Could you check a few things on this model? Use its own coordinates, in mm. A direction names the side the tool comes from. Round coordinates to 2 decimals unless told otherwise and drop trailing zeros. Loops run counter-clockwise (first coordinate to the right, second up) from the corner with the lowest first, then second, coordinate; pieces in that order, holes last. Notation, with made-up numbers: (22, -39) -> (39, -39) arc R13 ccw to (39, -18) -> close; hole circle Ø10 at (8, 18.5). An arc over 180 degrees is marked (long way). Put each result on its own line as item: value. Start each with the question number.
1. Which directions (+Z, -Z, +X, -X, +Y, -Y) give clear straight access to the entire face, cutting with the end or side of a thin tool? Please do faces 1 (the conical face through (-2.465, 114.221, -18.777)), 2 (the cylindrical face through (30.995, 18.783, 6.883)), 3 (the flat face through (0, 189.23, 0)).
2. I'm going to push flat-ended pins straight in: P1, Ø6, axis at y = 3, z = -4.5, coming from the +X side; P2, Ø1, axis at y = 116, z = -14.5, coming from the -X side; P3, Ø2, axis at x = -4.5, z = 21, coming from the -Y side. Where does each tip first touch, or does it pass through?
3. Imagine slicing it at A-A, the plane y = 167. Please give me the cut outline in (x, z), and give its area (3 significant figures).
4. If we mould it in two halves opening along Y, with no side actions, what happens to faces 4 (the cylindrical face through (-6.607, 23.091, 29.755)), 5 (the flat face through (0, 190.5, 0)), 6 (the flat face through (25, 38.1, 20)), 7 (the flat face through (-28.5, 39.37, 11.8))? For each: pulls with the +Y half, pulls with the -Y half, needs draft (parallel to the pull), parting line crosses it, or undercut.
5. I need wall thicknesses on line 1 (X direction, y = 26, z = 0); line 2 (Z direction, x = -12, y = 90.5). Which ranges of each line are inside material? Lowest first, please. Write a range as [from, to].
```python
from build123d import *

# Parameters (mm, degrees)
SKETCH1_R           = 31.75
BOSS_EXTRUDE1_DEPTH = 38.1
SKETCH2_R           = 33.734375
BOSS_EXTRUDE2_DEPTH = 152.4
BOSS_EXTRUDE2_TAPER = 11
FILLET1_R           = 2.794
SKETCH4_R           = 6.35
REVOLVE1_ANGLE      = 180
SKETCH5_R           = 31.75
BOSS_EXTRUDE3_DEPTH = 6.35


# Read off the part's stored shape, not the designer's step: Shell3
with BuildPart() as part:
    # Sketch1 → Boss-Extrude1 (new body)
    with BuildSketch(Plane(origin=(0, 0, 0), x_dir=(1, 0, 0), z_dir=(0, 1, 0))):
        with Locations(Location((0, 0, 0), (0, 0, 90))):
            Circle(SKETCH1_R)
    extrude(amount=BOSS_EXTRUDE1_DEPTH)

    # Sketch2 → Boss-Extrude2 (add)
    with BuildSketch(Plane(origin=(0, 38.1, 0), x_dir=(1, 0, 0), z_dir=(0, 1, 0))):
        Circle(SKETCH2_R)
    extrude(amount=BOSS_EXTRUDE2_DEPTH, taper=BOSS_EXTRUDE2_TAPER)

    # Fillet1
    fillet1_edges = [part.edges().sort_by_distance(p)[0] for p in [
        (-4.110815887, 190.5, 0),
    ]]
    fillet(fillet1_edges, radius=FILLET1_R)

    # Shell3 outline → Shell3 (revolve, cut)
    with BuildSketch(Plane.XY):
        with BuildLine():
            Line((32.193741805, 39.37), (3.303619853, 187.996792909))
            ThreePointArc((3.303619853, 187.996792909), (2.777003233, 188.881955865), (1.807620025, 189.23))
            Line((1.807620025, 189.23), (0, 189.23))
            Line((0, 189.23), (0, 1.27))
            Line((0, 1.27), (30.48, 1.27))
            Line((30.48, 1.27), (30.48, 39.37))
            Line((30.48, 39.37), (32.193741805, 39.37))
        make_face()
    revolve(axis=Axis((0, 0, 0), (0, 1, 0)), mode=Mode.SUBTRACT)

    # Sketch4 → Revolve1 (revolve)
    with BuildSketch(Plane.XZ):
        with Locations((-17.08043758, 0)):
            Circle(SKETCH4_R)
    revolve(axis=Axis((0, 0, 0), (0, 0, 1)), revolution_arc=REVOLVE1_ANGLE)

    # Sketch5 → Boss-Extrude3 (add)
    with BuildSketch(Plane.XZ):
        with Locations(Location((0, 0, 0), (0, 0, 270))):
            Circle(SKETCH5_R)
    extrude(amount=-BOSS_EXTRUDE3_DEPTH)


solid = part.part
```
Entries:
1. face 1: +Y
1. face 2: -Y
1. face 3: none
2. P1: x = 31.71
2. P2: x = -12.25
2. P3: y = 0
3. outline: circle Ø17.36 at (0, 0); hole circle Ø14.77 at (0, 0)
3. area: 65.3 mm^2
4. face 4: undercut
4. face 5: pulls with the +Y half
4. face 6: pulls with the -Y half
4. face 7: undercut
5. line 1: [-31.75, -30.48], [30.48, 31.75]
5. line 2: [-20.26, -18.74], [18.74, 20.26]
